```python
from build123d import *

# Parameters (mm, degrees)
SKETCH3_R               = 8
BOSS_EXTRUDE1_DEPTH     = 32.422105263
CUT_EXTRUDE1_DEPTH      = 12.326517504
CUT_EXTRUDE1_DEPTH_BACK = 12.326517504
BOSS_EXTRUDE2_DEPTH     = 1.2
CUT_EXTRUDE2_DEPTH      = 1.6
SKETCH8_R               = 1.4
SKETCH8_R_2             = 1.6
CUT_EXTRUDE3_DEPTH      = 2.64160469
CUT_EXTRUDE3_DEPTH_BACK = 36.765098388
CUT_EXTRUDE4_DEPTH      = 36.765098388


with BuildPart() as part:
    # Sketch3 → Boss-Extrude1 (new body)
    with BuildSketch(Plane(origin=(-20.344467381, 196.178792599, 0), x_dir=(-0.994665758, -0.103150523, 0), z_dir=(0.103150523, -0.994665758, 0))):
        with Locations((-10.431405186, 0)):
            Circle(SKETCH3_R)
    extrude(amount=BOSS_EXTRUDE1_DEPTH)

    # Sketch4 → Cut-Extrude1 (cut, two sides)
    with BuildSketch(Plane(origin=(10.375761543, 1.076004901, 0), x_dir=(0.103150523, -0.994665758, 0), z_dir=(-0.994665758, -0.103150523, 0))) as cut_extrude1_sk:
        Polygon((-197.230869842, 0), (-189.230869842, 8), (-197.230869842, 8), align=None)
        Polygon((-172.808764579, 8), (-164.808764579, 8), (-164.808764579, 0), align=None)
    extrude(amount=CUT_EXTRUDE1_DEPTH, mode=Mode.SUBTRACT)
    extrude(cut_extrude1_sk.sketch, amount=-CUT_EXTRUDE1_DEPTH_BACK, mode=Mode.SUBTRACT)

    # Sketch5 → Boss-Extrude2 (add, symmetric)
    with BuildSketch(Plane(origin=(10.375761543, 1.076004901, 0), x_dir=(0.103150523, -0.994665758, 0), z_dir=(-0.994665758, -0.103150523, 0))):
        with BuildLine():
            Line((-164.808764579, -2.8), (-162.383893448, 1.4))
            ThreePointArc((-162.383893448, 1.4), (-164.443291241, 2.776045612), (-166.788663566, 1.979898987))
            Line((-166.788663566, 1.979898987), (-164.808764579, 0))
            Line((-164.808764579, 0), (-164.808764579, -2.8))
        make_face()
    extrude(amount=BOSS_EXTRUDE2_DEPTH, both=True)

    # Sketch7 → Cut-Extrude2 (cut, symmetric)
    with BuildSketch(Plane(origin=(10.375761543, 1.076004901, 0), x_dir=(0.103150523, -0.994665758, 0), z_dir=(-0.994665758, -0.103150523, 0))):
        with BuildLine():
            Line((-194.968128142, 2.2627417), (-197.230869842, 0))
            Line((-197.230869842, 0), (-197.230869842, -3.2))
            ThreePointArc((-197.230869842, -3.2), (-194.274455338, -1.224586984), (-194.968128142, 2.2627417))
        make_face()
    extrude(amount=CUT_EXTRUDE2_DEPTH, both=True, mode=Mode.SUBTRACT)

    # Sketch8 → Cut-Extrude3 (cut, two sides)
    with BuildSketch(Plane(origin=(-20.344467381, 196.178792599, 0), x_dir=(0.994665758, 0.103150523, 0), z_dir=(-0.103150523, 0.994665758, 0))) as cut_extrude3_sk:
        with Locations((10.431405186, -5.5)):
            Circle(SKETCH8_R)
        with Locations((6.831405186, 3)):
            Circle(SKETCH8_R_2)
        with Locations((14.031405186, 3)):
            Circle(SKETCH8_R_2)
    extrude(amount=CUT_EXTRUDE3_DEPTH, mode=Mode.SUBTRACT)
    extrude(cut_extrude3_sk.sketch, amount=-CUT_EXTRUDE3_DEPTH_BACK, mode=Mode.SUBTRACT)

    # Sketch9 → Cut-Extrude4 (cut, through all)
    with BuildSketch(Plane(origin=(-20.344467381, 196.178792599, 0), x_dir=(0.994665758, 0.103150523, 0), z_dir=(-0.103150523, 0.994665758, 0))):
        with BuildLine():
            Line((7.933405986, 7.6), (12.929404385, 7.6))
            ThreePointArc((12.929404385, 7.6), (10.431405186, 8), (7.933405986, 7.6))
        make_face()
        with BuildLine():
            Line((7.933405986, -7.6), (12.929404385, -7.6))
            ThreePointArc((12.929404385, -7.6), (10.431405186, -8), (7.933405986, -7.6))
        make_face()
    extrude(amount=-CUT_EXTRUDE4_DEPTH, mode=Mode.SUBTRACT)


solid = part.part
```
For this review, take the finished solid that the model builds, in its own axes (mm). A direction names the side the tool comes from. Round coordinates to 2 decimals unless told otherwise and drop trailing zeros. Write each loop counter-clockwise with the first axis right and the second up, starting at its lowest first coordinate (ties: lowest second). Pieces come first, ordered by that corner, then holes. Notation, with made-up numbers: (59, 88.5) -> (83, 88.5) arc R4 ccw to (83, 92.5) -> close; hole circle Ø4 at (55, 22). An arc over 180 degrees is marked (long way). Use one line per item in the form item = value.
Q1. Consider section D-D (z = -6.5). State the section outline as (x, y) points, then the cut area to 3 significant figures.
Resolved:
outline = (-14.61, 196.77) -> (-11.26, 164.52) -> (-1.99, 165.49) -> (-5.33, 197.74) -> close
area = 302 mm²
Q2. Machinability: for faces 1 (the flat face through (-5.41, 164.94, 0.66)), 2 (the flat face through (-8.215, 195.851, -0.43)), 3 (the cylindrical face through (-0.71, 182.15, -2.33)), which of the approach directions +Z, -Z, +X, -X, +Y, -Y give a long, thin tool a straight path to every point of the face, cutting with its end or side? Answer none if there is none.
Resolved:
face_1 = +Z, +X
face_2 = none
face_3 = +X, +Y
Q3. The part is to be moulded in two halves that separate along Y. For faces 4 (the flat face through (-11.397, 195.521, -0.43)), 5 (the flat face through (-7.8, 164.7, 0.7)), 6 (the cylindrical face through (-8.497, 181.297, 4.112)), say which applies: released by +Y, released by -Y, zero draft, split by the parting line, or undercut.
Resolved:
face_4 = released by +Y
face_5 = released by -Y
face_6 = undercut
Q4. To check wall thickness, follow probe 1 along X at (y, z) = (182, -3); probe 2 along X at (y, z) = (181, -2.25); probe 3 along Z at (x, y) = (-5, 170). State the ranges of each line that lie inside material, in increasing order. Write a range as from..to.
Resolved:
probe_1 = -15.84..-13.61, -10.4..-6.38, -3.16..-0.93
probe_2 = -16..-13.32, -10.48..-6.08, -3.24..-0.56
probe_3 = -7.6..-3.63, -2.37..4.8
Q5. Consider section B-B (y = 169.5). State how many separate pieces and enclosed holes the cut face has, then the cut area to 3 significant figures.
Resolved:
separate_pieces = 1
enclosed_holes = 2
area = 151 mm²
Q6. Clearance check with flat-ended pins moving along their axes: pin 1 Ø2 at (x, z) = (-12.5, 0.5) entering from +Y; pin 2 Ø4 at (x, z) = (-6, -4.5) entering from +Y; pin 3 Ø3 at (x, y) = (-3, 191) entering from +Z. State where each tip first meets the part, or that it passes through.
Resolved:
pin_1 = 197.08
pin_2 = 197.87
pin_3 = 6.41
Q7. Consider section A-A (z = -2). State the section outline as (x, y) points.
Resolved:
outline = (-17.67, 196.46) -> (-14.33, 164.21) -> (-11.45, 164.51) -> (-14.79, 196.75) -> close; (-12.31, 197.01) -> (-8.96, 164.76) -> (-7.82, 164.88) -> (-7.77, 164.42) -> (-5.38, 164.67) -> (-5.43, 165.13) -> (-4.29, 165.25) -> (-7.63, 197.5) -> (-8.38, 197.42) -> (-8.12, 194.94) -> (-11.3, 194.61) -> (-11.56, 197.09) -> close; (-5.15, 197.75) -> (-1.8, 165.51) -> (1.08, 165.8) -> (-2.26, 198.05) -> close
